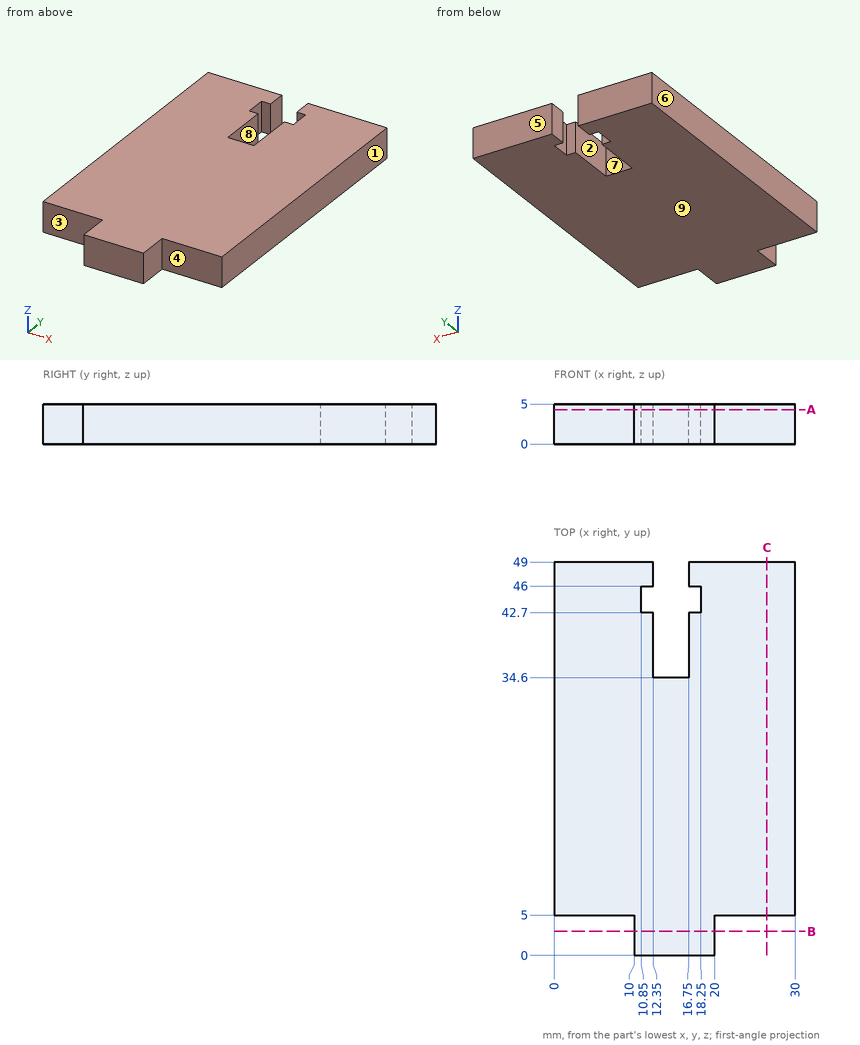
Input: dimensioned drawing with shaded views. Units: mm. Origin: part minimum x, y, z. A direction names the side the tool comes from. Give positions to 0.01 mm unless a question says otherwise; leave off trailing zeros. Write each loop counter-clockwise with the first axis right and the second up, starting at its lowest first coordinate (ties: lowest second). Pieces come first, ordered by that corner, then holes.
Q1. Section A-A, the plane z = 4.3. Output: boundary loops of the cut face in (x, y).
Q2. Section C-C, the plane x = 26.5. Output: boundary loops of the cut face in (y, z).
Q3. Set-up query: the marked faces 1, 2, 3, 4 and 5. Return all of +Z, -Z, +X, -X, +Y, -Y with unobstructed straight access to the full face (end or side cutting, diameter ignored); none if empty.
Q4. Material intervals for probe 1 along X at (y, z) = (35.5, 2.8); probe 2 along Y at (x, z) = (11.5, 1); probe 3 along Y at (x, z) = (6.25, 3.25), sorted ascending.
Q5. Section B-B, the plane y = 3. Output: boundary loops of the cut face in (x, z), plus the area to 3 significant figures.
Q6. First-contact query: P1, Ø1.5, axis at y = 1.5, z = 2.5, coming from the -X side. Flat tip, straight axial feed; report the tip coordinate or a pass-through.
Q7. Pull-direction query (X, two-part tool) for the marked faces 6, 7, 8 and 9; classes: pulls with the +X half, pulls with the -X half, needs draft (parallel to the pull), parting line crosses it, or undercut.
Filled in:
1. outline: (0, 5) - (10, 5) - (10, 0) - (20, 0) - (20, 5) - (30, 5) - (30, 49) - (16.75, 49) - (16.75, 46) - (18.25, 46) - (18.25, 42.7) - (16.75, 42.7) - (16.75, 34.6) - (12.35, 34.6) - (12.35, 42.7) - (10.85, 42.7) - (10.85, 46) - (12.35, 46) - (12.35, 49) - (0, 49) - close
2. outline: (5, 0) - (49, 0) - (49, 5) - (5, 5) - close
3. face 1: +Z, -Z, +X, +Y, -Y
3. face 2: +Z, -Z, +Y
3. face 3: +Z, -Z, -X, -Y
3. face 4: +Z, -Z, +X, -Y
3. face 5: +Z, -Z, +X, -X, +Y
4. probe 1: x = 0 to 12.35, 16.75 to 30
4. probe 2: y = 0 to 42.7, 46 to 49
4. probe 3: y = 5 to 49
5. outline: (10, 0) - (20, 0) - (20, 5) - (10, 5) - close
5. area: 50.0 mm2
6. P1: stops at x = 10
7. face 6: pulls with the -X half
7. face 7: undercut
7. face 8: undercut
7. face 9: needs draft
